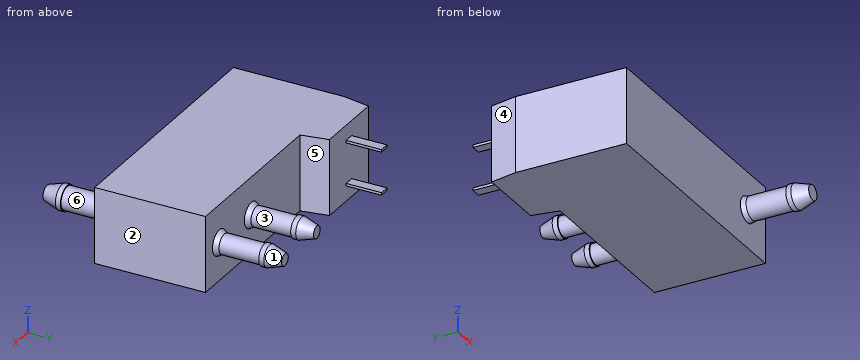
```python
from build123d import *

# Parameters (mm, degrees)
SKETCH1_W                       = 50
SKETCH1_H                       = 22
BOSS_EXTRUDE1_DEPTH             = 7.5
BOSS_EXTRUDE3_REACH             = 30.324
BOSS_EXTRUDE3_DIRECTION_2_REACH = 30.324
SKETCH9_W                       = 2
SKETCH9_H                       = 0.5
BOSS_EXTRUDE4_DEPTH             = 7


with BuildPart() as part:
    # Sketch1 → Boss-Extrude1 (new, symmetric)
    with BuildSketch(Plane.XY):
        Rectangle(SKETCH1_W, SKETCH1_H)
    extrude(amount=BOSS_EXTRUDE1_DEPTH, both=True)

    # Boss-Extrude3: up to this face of the body (flat: up to its plane)
    boss_extrude3_end = Plane(part.part.faces().sort_by_distance((0, 0, 7.5))[0])
    # Sketch3 → Boss-Extrude3 (add, up to the picked face)
    with BuildSketch(Plane.XY, mode=Mode.PRIVATE) as boss_extrude3_sk1:
        Polygon((-25, 11), (-24, 16.31597155), (-10, 16.31597155), (-9, 11), align=None)
    boss_extrude3_tool1 = split(extrude(boss_extrude3_sk1.sketch, amount=BOSS_EXTRUDE3_REACH, mode=Mode.PRIVATE), bisect_by=boss_extrude3_end, keep=Keep.BOTH, mode=Mode.PRIVATE)
    add(boss_extrude3_tool1.solids().sort_by(Axis((-17, 13.598919, 0), (0, 0, 1)))[0])

    # Boss-Extrude3 direction 2: up to this face of the body (flat: up to its plane)
    boss_extrude3_direction_2_end = Plane(part.part.faces().sort_by_distance((0, 0, -7.5))[0])
    # Sketch3 → Boss-Extrude3 direction 2 (add, up to the picked face)
    with BuildSketch(Plane.XY, mode=Mode.PRIVATE) as boss_extrude3_direction_2_sk1:
        Polygon((-25, 11), (-24, 16.31597155), (-10, 16.31597155), (-9, 11), align=None)
    boss_extrude3_direction_2_tool1 = split(extrude(boss_extrude3_direction_2_sk1.sketch, amount=-BOSS_EXTRUDE3_DIRECTION_2_REACH, mode=Mode.PRIVATE), bisect_by=boss_extrude3_direction_2_end, keep=Keep.BOTH, mode=Mode.PRIVATE)
    add(boss_extrude3_direction_2_tool1.solids().sort_by(Axis((-17, 13.598919, 0), (0, 0, -1)))[0])

    # Sketch5 → Revolve1 (revolve)
    with BuildSketch(Plane.XY, mode=Mode.PRIVATE) as revolve1_sk:
        Polygon((8.5, 11), (11, 11), (10.474759089, 12), (10.474759089, 20), (10.674759089, 20), (10.674759089, 21), (9.7, 24), (8.5, 24), align=None)
    revolve(revolve1_sk.sketch.rotate(Axis((8.5, 24, 0), (0, -1, 0)), 90), axis=Axis((8.5, 24, 0), (0, -1, 0)))

    # Sketch6 → Revolve2 (revolve)
    with BuildSketch(Plane.XY, mode=Mode.PRIVATE) as revolve2_sk:
        Polygon((20, 11), (22.5, 11), (21.974759089, 12), (21.974759089, 20), (22.174759089, 20), (22.174759089, 21), (21.2, 24), (20, 24), align=None)
    revolve(revolve2_sk.sketch.rotate(Axis((20, 24, 0), (0, -1, 0)), 90), axis=Axis((20, 24, 0), (0, -1, 0)))

    # Sketch8 → Revolve3 (revolve)
    with BuildSketch(Plane.XY, mode=Mode.PRIVATE) as revolve3_sk:
        Polygon((18.5, -11), (18.5, -24), (17, -24), (16.025240911, -21), (16.025240911, -20), (16.225240911, -20), (16.225240911, -12), (16, -11), align=None)
    revolve(revolve3_sk.sketch.rotate(Axis((18.5, -11, 0), (0, -1, 0)), 270), axis=Axis((18.5, -11, 0), (0, -1, 0)))

    # Sketch9 → Boss-Extrude4 (add)
    with BuildSketch(Plane(origin=(0, 16.31597155, 0), x_dir=(1, 0, 0), z_dir=(0, 1, 0))):
        with Locations((-17, 4.25)):
            Rectangle(SKETCH9_W, SKETCH9_H)
    boss_extrude4 = extrude(amount=BOSS_EXTRUDE4_DEPTH)

    # Mirror1: Boss-Extrude4 across plane
    add(boss_extrude4.mirror(Plane.XY))


solid = part.part
```
Geometry: final body of the model. Coordinates: model frame, mm. Face numbers are marked on the shaded views. A direction names the side the tool comes from. Coordinates: 2 decimals unless noted, no trailing zeros. Loops run counter-clockwise (first coordinate to the right, second up) from the corner with the lowest first, then second, coordinate; pieces in that order, holes last. Notation, with made-up numbers: (-38, -20) -> (-27, -20) arc R16 ccw to (-27, -5) -> close; hole circle Ø11 at (33.5, 19). An arc over 180 degrees is marked (long way). Use a Markdown table: item, result. Add a question column.
(1) Section query D-D, the plane y = -18. Return loops of the section in (x, z).
(2) Mould query, pull axis Y, two halves, no side actions, for the marked faces 1, 2 and 3. Classes: pulls with the +Y half, pulls with the -Y half, needs draft (parallel to the pull), parting line crosses it, or undercut.
(3) Section query C-C, the plane z = -6. Return loops of the section in (x, y).
(4) Pin query (flat end, axial travel): pin 1 Ø1.6 at (x, y) = (-17, 21.5) entering from -Z; pin 2 Ø1 at (x, y) = (-16.5, 18.5) entering from +Z; pin 3 Ø5.5 at (x, z) = (18, 0) entering from +Y; pin 4 Ø2 at (x, z) = (-4, 0.5) entering from -Y. Return the tip coordinate at first contact, or that it passes through.
(5) Access query for the marked faces 4, 5 and 6. Directions: +Z, -Z, +X, -X, +Y, -Y. A direction counts if a zero-diameter tool reaches every point of the face in a straight line with its end or side. Return the directions, or none.
(6) Line query: line 1 along Y through (x, z) = (-11, -0.5); line 2 along Y through (x, z) = (-6.5, 3); line 3 along X through (y, z) = (21.5, 1). Output: solid intervals per line, ascending.
(7) Section query B-B, the plane x = 8.5. Return loops of the section in (y, z), plus the area to 3 significant figures.
(8) Section query A-A, the plane y = 17. Return loops of the section in (x, z), plus the area to 3 significant figures.
Answer:
| question | item | result |
|---|---|---|
| 1 | outline | circle Ø4.55 at (18.5, 0) |
| 2 | face 1 | pulls with the +Y half |
| 2 | face 2 | needs draft |
| 2 | face 3 | undercut |
| 3 | outline | (-25, -11) -> (25, -11) -> (25, 11) -> (-9, 11) -> (-10, 16.32) -> (-24, 16.32) -> (-25, 11) -> close |
| 4 | pin 1 | stops at z = -4.5 |
| 4 | pin 2 | stops at z = 4.5 |
| 4 | pin 3 | stops at y = 24 |
| 4 | pin 4 | stops at y = -11 |
| 5 | face 4 | +Z, -Z, -X, +Y |
| 5 | face 5 | +Z, -Z, +Y |
| 5 | face 6 | none |
| 6 | line 1 | y = -11 to 16.32 |
| 6 | line 2 | y = -11 to 11 |
| 6 | line 3 | x = 6.75 to 10.25, 18.25 to 21.75 |
| 7 | outline | (-11, -7.5) -> (11, -7.5) -> (11, -2.5) -> (12, -1.97) -> (20, -1.97) -> (20, -2.17) -> (21, -2.17) -> (24, -1.2) -> (24, 1.2) -> (21, 2.17) -> (20, 2.17) -> (20, 1.97) -> (12, 1.97) -> (11, 2.5) -> (11, 7.5) -> (-11, 7.5) -> close |
| 7 | area | 381 mm^2 |
| 8 | outline | (-18, -4.5) -> (-16, -4.5) -> (-16, -4) -> (-18, -4) -> close; (-18, 4) -> (-16, 4) -> (-16, 4.5) -> (-18, 4.5) -> close; circle Ø3.95 at (8.5, 0); circle Ø3.95 at (20, 0) |
| 8 | area | 26.5 mm^2 |
